```python
from build123d import *

# Parameters (mm, degrees)
F0_W     = 20.1
F0_H     = 10.1
F0_W_2   = 10.1
F0_H_2   = 20.1
F1_DEPTH = 5
F2_DEPTH = 2.1
F3_D     = 3
F5_DEPTH = 2.5
F6_R     = 0.5


with BuildPart() as f1:
    # F0 (on Top) → F1 (new body)
    with BuildSketch(Plane.XY):
        Polygon((0, 50), (0, 0), (50, 0), (50, 14), (42, 14), (14, 14), (14, 42), (14, 50), align=None)
        with Locations((28.5, 6.05)):
            Rectangle(F0_W, F0_H, mode=Mode.SUBTRACT)
        with Locations((6.05, 28.5)):
            Rectangle(F0_W_2, F0_H_2, mode=Mode.SUBTRACT)
        Polygon((42, 14), (50, 14), (14, 50), (14, 42), align=None)
        with Locations((6.05, 28.5)):
            Rectangle(F0_W_2, F0_H_2)
        with Locations((28.5, 6.05)):
            Rectangle(F0_W, F0_H)
    extrude(amount=F1_DEPTH)

    # F0 (on Top) → F2 (cut)
    with BuildSketch(Plane.XY):
        with Locations((6.05, 28.5)):
            Rectangle(F0_W_2, F0_H_2)
        with Locations((28.5, 6.05)):
            Rectangle(F0_W, F0_H)
    extrude(amount=F2_DEPTH, mode=Mode.SUBTRACT)

    # F3 (through all)
    with Locations(Plane(origin=(0, 0, 0), x_dir=(1, 0, 0), z_dir=(0, 0, -1))):
        with Locations((7, -15), (15, -7), (42, -7), (7, -42)):
            Hole(F3_D / 2)

    # F4 (on face) → F5 (cut)
    with BuildSketch(Plane.XY.offset(5)):
        Polygon((7, 45.3486315613), (4.1, 43.6743157806), (4.1, 40.3256842194), (7, 38.6513684387), (9.9, 40.3256842194), (9.9, 43.6743157806), align=None)
        Polygon((7, 18.3486315613), (4.1, 16.6743157806), (4.1, 13.3256842194), (7, 11.6513684387), (9.9, 13.3256842194), (9.9, 16.6743157806), align=None)
        Polygon((18.3486315613, 7), (16.6743157806, 9.9), (13.3256842194, 9.9), (11.6513684387, 7), (13.3256842194, 4.1), (16.6743157806, 4.1), align=None)
        Polygon((40.3256842194, 9.9), (38.6513684387, 7), (40.3256842194, 4.1), (43.6743157806, 4.1), (45.3486315613, 7), (43.6743157806, 9.9), align=None)
    extrude(amount=-F5_DEPTH, mode=Mode.SUBTRACT)

    # F6
    f6_edges = [f1.edges().sort_by_distance(p)[0] for p in [
        (0, 0, 2.5),
        (50, 0, 2.5),
        (50, 14, 2.5),
        (14, 50, 2.5),
        (0, 50, 2.5),
        (0, 25, 5),
        (7, 50, 0),
        (32, 32, 0),
        (50, 7, 0),
        (25, 0, 0),
        (28, 14, 0),
        (28, 28, 0),
        (14, 28, 0),
        (0, 25, 0),
        (25, 0, 5),
        (50, 7, 5),
        (32, 32, 5),
        (14, 28, 5),
        (28, 28, 5),
        (28, 14, 5),
        (7, 50, 5),
    ]]
    fillet(f6_edges, radius=F6_R)


solid = f1.part
```
For this review, take the finished solid that the model builds, in its own axes (mm). A direction names the side the tool comes from. Round coordinates to 2 decimals unless told otherwise and drop trailing zeros. Loops run counter-clockwise (first coordinate to the right, second up) from the corner with the lowest first, then second, coordinate; pieces in that order, holes last.
Q1. Mouldability with a two-part tool opening along X and no side actions: class faces 1 (the face through (31.64, 32.14, 0.14)), 2 (the face through (0, 25, 2)), 3 (the face through (28, 1, 1)) as +X half, -X half, draft (parallel to the pull), parting line (faces both ways), or undercut.
Result sheet:
face 1: +X half
face 2: -X half
face 3: undercut
Q2. To check wall thickness, follow line 1 along X through (y, z) = (7, 1); line 2 along Y through (x, z) = (15, 1.45). State the ranges of each line that lie inside material, in increasing order.
Result sheet:
line 1: x = 0 to 13.5, 16.5 to 18.45, 38.55 to 40.5, 43.5 to 50
line 2: y = 0 to 5.5, 8.5 to 14, 41 to 49
Q3. Machinability: for faces 4 (the face through (39.477, 5.57, 3.768)), 5 (the face through (6, 29, 2.1)), 6 (the face through (32, 32, 2)), which of the approach directions +Z, -Z, +X, -X, +Y, -Y give a long, thin tool a straight path to every point of the face, cutting with its end or side? Answer none if there is none.
Result sheet:
face 4: +Z
face 5: -Z
face 6: +Z, -Z, +X, +Y
Q4. Add section A-A on y = 10.5. Write out the cut boundary in (x, z), plus the area to 3 significant figures.
Result sheet:
outline: (0, 0.5) arc R0.5 ccw to (0.5, 0) - (18.45, 0) - (18.45, 2.1) - (38.55, 2.1) - (38.55, 0) - (49.5, 0) arc R0.5 ccw to (50, 0.5) - (50, 4.5) arc R0.5 ccw to (49.5, 5) - (0.5, 5) arc R0.5 ccw to (0, 4.5) - close
area: 208 mm2
Q5. Insertion check: pin 1 Ø1.2 at (x, z) = (14.5, 3) entering from +Y; pin 2 Ø3 at (x, y) = (42, 6) entering from +Z; pin 3 Ø2 at (x, z) = (41.5, 3.5) entering from +Y. Each pin has a flat end and moves straight along its axis. Give the tip position at first contact, or say it passes through.
Result sheet:
pin 1: stops at y = 49.99
pin 2: stops at z = 2.5
pin 3: stops at y = 23.5
Q6. Add section B-B on z = 3.9. Give the number of separate pieces and of enclosed holes in the cut face, plus the area to 3 significant figures.
Result sheet:
separate pieces: 1
enclosed holes: 5
area: 1,340 mm2
Q7. Add section C-C on x = 12.5. Write out the cut boundary in (y, z).
Result sheet:
outline: (0, 0.5) arc R0.5 ccw to (0.5, 0) - (49.5, 0) arc R0.5 ccw to (50, 0.5) - (50, 4.5) arc R0.5 ccw to (49.5, 5) - (8.47, 5) - (8.47, 2.5) - (5.53, 2.5) - (5.53, 5) - (0.5, 5) arc R0.5 ccw to (0, 4.5) - close
